```python
from build123d import *

# Parameters (mm, degrees)
BOSS_EXTRUDE1_DEPTH   = 5.08
LPATTERN1_COUNT       = 2
LPATTERN1_PITCH       = 104.14
SKETCH2_R             = 6.35
BOSS_EXTRUDE2_DEPTH   = 104.14
LPATTERN2_COUNT       = 3
LPATTERN2_PITCH       = 114.3
BODY_MOVE_COPY1_ANGLE = 120
BODY_MOVE_COPY2_ANGLE = 120
SKETCH3_R             = 12.7
BOSS_EXTRUDE3_DEPTH   = 5.08
BOSS_EXTRUDE4_START   = 114.3
SKETCH3_2_R           = 12.7
BOSS_EXTRUDE4_DEPTH   = 5.08
SKETCH4_R             = 6.985
BOSS_EXTRUDE5_DEPTH   = 76.2
SKETCH5_R             = 6.35
BOSS_EXTRUDE6_DEPTH   = 76.2
BOSS_EXTRUDE8_START   = 5.499261
SKETCH6_W             = 6.35
SKETCH6_H             = 25.4
BOSS_EXTRUDE8_DEPTH   = 4.660739


with BuildPart() as part:
    # Sketch1 → Boss-Extrude1 (new body)
    with BuildSketch(Plane.XY):
        with BuildLine():
            ThreePointArc((21.401887456, 5.241250721), (16.887307357, 9.873763366), (15.24, 16.129))
            Line((15.24, 16.129), (15.24, 34.919226796))
            ThreePointArc((15.24, 34.919226796), (0, 38.1), (-15.24, 34.919226796))
            Line((-15.24, 34.919226796), (-15.24, 16.129))
            ThreePointArc((-15.24, 16.129), (-16.887307357, 9.873763366), (-21.401887456, 5.241250721))
            ThreePointArc((-21.401887456, 5.241250721), (-21.59, 5.130477372), (-21.779988806, 5.022953805))
            Line((-21.779988806, 5.022953805), (-37.860937485, -4.261386244))
            ThreePointArc((-37.860937485, -4.261386244), (0, -38.1), (37.860937485, -4.261386244))
            Line((37.860937485, -4.261386244), (21.779988806, 5.022953805))
            ThreePointArc((21.779988806, 5.022953805), (21.59, 5.130477372), (21.401887456, 5.241250721))
        make_face()
    extrude(amount=-BOSS_EXTRUDE1_DEPTH)


with BuildPart() as lpattern1_1:
    # LPattern1: pattern copy
    add(part.part.moved(Location(Vector(0, 0, -1) * (1 * LPATTERN1_PITCH))))


with BuildPart() as part_1:
    add(part.part)

    add(lpattern1_1.part)  # Boss-Extrude2 merges LPattern1_1
    # Sketch2 → Boss-Extrude2 (add)
    with BuildSketch(Plane(origin=(0, 0, -5.08), x_dir=(-1, 0, 0), z_dir=(0, 0, -1))):
        with Locations((0, 25.4)):
            Circle(SKETCH2_R)
    extrude(amount=BOSS_EXTRUDE2_DEPTH)


with BuildPart() as lpattern2_1:
    # LPattern2: pattern copy
    add(part_1.part.moved(Location(Vector(0, 0, -1) * (1 * LPATTERN2_PITCH))))


with BuildPart() as lpattern2_2:
    # LPattern2: pattern copy
    add(part_1.part.moved(Location(Vector(0, 0, -1) * (2 * LPATTERN2_PITCH))))


with BuildPart() as lpattern2_1_1:
    # Body-Move/Copy1: moved
    add(lpattern2_1.part.rotate(Axis((0, 0, 0), (0, 0, 1)), BODY_MOVE_COPY1_ANGLE))


with BuildPart() as lpattern2_2_1:
    # Body-Move/Copy2: moved
    add(lpattern2_2.part.rotate(Axis((0, 0, 0), (0, 0, -1)), BODY_MOVE_COPY2_ANGLE))


with BuildPart() as part_2:
    add(part_1.part)

    add(lpattern2_1_1.part)  # Boss-Extrude3 merges LPattern2_1
    # Sketch3 → Boss-Extrude3 (add)
    with BuildSketch(Plane(origin=(0, 0, -109.22), x_dir=(-1, 0, 0), z_dir=(0, 0, -1))):
        Circle(SKETCH3_R)
    extrude(amount=BOSS_EXTRUDE3_DEPTH)

    add(lpattern2_2_1.part)  # Boss-Extrude4 merges LPattern2_2
    # Sketch3<2> → Boss-Extrude4 (add)
    with BuildSketch(Plane(origin=(0, 0, -109.22), x_dir=(-1, 0, 0), z_dir=(0, 0, -1)).offset(BOSS_EXTRUDE4_START)):
        Circle(SKETCH3_2_R)
    extrude(amount=BOSS_EXTRUDE4_DEPTH)

    # Sketch4 → Boss-Extrude5 (add)
    with BuildSketch(Plane(origin=(0, 0, -337.82), x_dir=(-1, 0, 0), z_dir=(0, 0, -1))):
        Circle(SKETCH4_R)
    extrude(amount=BOSS_EXTRUDE5_DEPTH)

    # Sketch5 → Boss-Extrude6 (add)
    with BuildSketch(Plane.XY):
        Circle(SKETCH5_R)
    extrude(amount=BOSS_EXTRUDE6_DEPTH)

    # Sketch6 → Boss-Extrude8 (add)
    with BuildSketch(Plane(origin=(0, 0, 0), x_dir=(1, 0, 0), z_dir=(0, 1, 0)).offset(BOSS_EXTRUDE8_START)):
        with Locations((0, -57.15)):
            Rectangle(SKETCH6_W, SKETCH6_H)
    extrude(amount=BOSS_EXTRUDE8_DEPTH)


solid = part_2.part
```
Geometry: final body of the model. Coordinates: model frame, mm. A direction names the side the tool comes from. Give positions to 0.01 mm unless a question says otherwise; leave off trailing zeros. Loops run counter-clockwise (first coordinate to the right, second up) from the corner with the lowest first, then second, coordinate; pieces in that order, holes last. Notation, with made-up numbers: (11.5, 23.5) -> (49.5, 23.5) arc R10 cw to (49.5, 38.5) -> close; hole circle Ø10 at (-23, -24). An arc over 180 degrees is marked (long way). Use CSV: the item, a comma, the result in double quotes.
(1) First-contact query: P1, Ø20.5, axis at x = 15, y = -2, coming from the -Z side; P2, Ø10, axis at x = 7, z = -336.5, coming from the +Y side; P3, Ø12, axis at y = 25.5, z = -88, coming from the +X side; P4, Ø2, axis at x = 17.5, y = 26.5, coming from the +Z side. Flat tips, straight axial feed; report the tip coordinate or a pass-through.
From the geometry:
P1,"z = -414.02"
P2,"y = 38.05"
P3,"x = 6.35"
P4,"z = -114.3"
(2) Ray query, line 1 along Z through (x, y) = (-2.5, -18); line 2 along Z through (x, y) = (-3, -0.5); line 3 along Z through (x, y) = (-4, -8). Return the intervals inside material, ascending. Write a range as [from, to].
From the geometry:
line 1,"[-337.82, -332.74], [-233.68, -228.6], [-223.52, -218.44], [-119.38, -114.3], [-109.22, -104.14], [-5.08, 0]"
line 2,"[-414.02, -332.74], [-233.68, -218.44], [-119.38, -104.14], [-5.08, 76.2]"
line 3,"[-337.82, -332.74], [-233.68, -218.44], [-119.38, -104.14], [-5.08, 0]"
(3) Access query for faces 5 (the face through (29.84, 0.37, -335.24)), 6 (the face through (29.933, 0.316, -106.644)), 7 (the face through (2.75, -12.4, -111.72)). Directions: +Z, -Z, +X, -X, +Y, -Y. A direction counts if a zero-diameter tool reaches every point of the face in a straight line with its end or side. Return the directions, or none.
From the geometry:
face 5,"-Z, +X, +Y"
face 6,"+Z, +X, +Y"
face 7,"none"
(4) Cut plane A-A (y = 0). Count the separate pieces of the cut face and the enclosed holes in it, plus the area to 3 significant figures.
From the geometry:
separate pieces,"4"
enclosed holes,"0"
area,"4,300 mm^2"
(5) Cut plane B-B (z = -95.5). Output: boundary loops of the cut face in (x, y).
From the geometry:
outline,"circle Ø12.7 at (0, 25.4)"
(6) Cut plane C-C (z = -370). Output: boundary loops of the cut face in (x, y) (3 decimals), plus the area to 3 significant figures.
From the geometry:
outline,"circle Ø13.97 at (0, 0)"
area,"153 mm^2"
(7) Pull-direction query (Z, two-part tool) for faces 1 (the face through (0, 0, -414.02)), 2 (the face through (14, 8, -223.52)), 3 (the face through (-29.708, 0.446, -106.644)), 4 (the face through (0, 0, 76.2)); classes: released by +Z, released by -Z, zero draft, split by the parting line, or undercut.
From the geometry:
face 1,"released by -Z"
face 2,"undercut"
face 3,"zero draft"
face 4,"released by +Z"
